```python
from build123d import *

# Parameters (mm, degrees)
SKETCH001_W   = 141
SKETCH001_H   = 55
PAD_DEPTH     = 3.6
SKETCH002_R   = 5
SKETCH002_R_2 = 1.6
PAD001_DEPTH  = 2
SKETCH003_R   = 1
POCKET_DEPTH  = 1.601


with BuildPart() as part:
    # Sketch001 → Pad (new body)
    with BuildSketch(Plane.XY):
        with BuildLine():
            Line((0, -3), (141, -3))
            ThreePointArc((141, -3), (143.12132, -2.12132), (144, 0))
            Line((144, 0), (144, 55))
            ThreePointArc((144, 55), (143.12132, 57.12132), (141, 58))
            Line((141, 58), (0, 58))
            ThreePointArc((0, 58), (-2.12132, 57.12132), (-3, 55))
            Line((-3, 55), (-3, 0))
            ThreePointArc((-3, 0), (-2.12132, -2.12132), (0, -3))
        make_face()
        with Locations((70.5, 27.5)):
            Rectangle(SKETCH001_W, SKETCH001_H, mode=Mode.SUBTRACT)
    extrude(amount=PAD_DEPTH)

    # Sketch002 → Pad001 (join)
    with BuildSketch(Plane.XY):
        with Locations((3.19, 34.92)):
            Circle(SKETCH002_R)
        with Locations((3.19, 34.92)):
            Circle(SKETCH002_R_2, mode=Mode.SUBTRACT)
        with Locations((3.19, 4.44)):
            Circle(SKETCH002_R)
        with Locations((3.19, 4.44)):
            Circle(SKETCH002_R_2, mode=Mode.SUBTRACT)
        with Locations((137.81, 4.44)):
            Circle(SKETCH002_R)
        with Locations((137.81, 4.44)):
            Circle(SKETCH002_R_2, mode=Mode.SUBTRACT)
        with Locations((137.81, 34.92)):
            Circle(SKETCH002_R)
        with Locations((137.81, 34.92)):
            Circle(SKETCH002_R_2, mode=Mode.SUBTRACT)
    extrude(amount=PAD001_DEPTH)

    # Sketch003 → Pocket (cut, through all)
    with BuildSketch(Plane.XY.offset(2)):
        with Locations((0, 55)):
            Circle(SKETCH003_R)
        with Locations((141, 55)):
            Circle(SKETCH003_R)
        Circle(SKETCH003_R)
        with Locations((141, 0)):
            Circle(SKETCH003_R)
    extrude(amount=POCKET_DEPTH, mode=Mode.SUBTRACT)


solid = part.part
```
Work out the finished part from the listing and answer in its coordinate system (mm). A direction names the side the tool comes from. Give positions to 0.01 mm unless a question says otherwise; leave off trailing zeros. Order: outer loops, then holes, each group sorted by start corner. A loop starts at its lowest first (then second) coordinate and runs counter-clockwise, first axis right, second up.
1. This flat-tipped pin is pushed along its axis until it touches: P1, Ø5, axis at x = 3.19, y = 34.92, coming from the +Z side. Where does it stop, or does it pass through?
Result sheet:
P1: stops at z = 2
2. The mould has two halves that part along X. Classify faces 1 (the flat face through (-3, 28, 2)), 2 (the flat face through (144, 27, 2)), 3 (the flat face through (70, 0, 2)), 4 (the flat face through (5, 35, 2)): released by +X, released by -X, zero draft, split by the parting line, or undercut.
Result sheet:
face 1: released by -X
face 2: released by +X
face 3: undercut
face 4: undercut
3. Section B-B, the plane y = 14 is taken. Determine the outline of the cut face in (x, z), and give its area (3 significant figures).
Result sheet:
outline: (-3, 0) - (0, 0) - (0, 3.6) - (-3, 3.6) - close; (141, 0) - (144, 0) - (144, 3.6) - (141, 3.6) - close
area: 21.6 mm2
4. For faces 5 (the cylindrical face through (143.1, -2.14, 1.77)), 6 (the flat face through (5, 5, 2)), 7 (the flat face through (70, 55, 2)), determine the directions among +Z, -Z, +X, -X, +Y, -Y from which every point of the face is accessible in a straight line to the end or side of a thin tool.
Result sheet:
face 5: +Z, -Z, +X, -Y
face 6: +Z
face 7: +Z, -Z
5. Section C-C, the plane x = 34.5 is taken. Determine the outline of the cut face in (y, z), and give its area (3 significant figures).
Result sheet:
outline: (-3, 0) - (0, 0) - (0, 3.6) - (-3, 3.6) - close; (55, 0) - (58, 0) - (58, 3.6) - (55, 3.6) - close
area: 21.6 mm2
6. Section A-A, the plane x = 3.19 is taken. Determine the outline of the cut face in (y, z).
Result sheet:
outline: (-3, 0) - (2.84, 0) - (2.84, 2) - (0, 2) - (0, 3.6) - (-3, 3.6) - close; (6.04, 0) - (9.44, 0) - (9.44, 2) - (6.04, 2) - close; (29.92, 0) - (33.32, 0) - (33.32, 2) - (29.92, 2) - close; (36.52, 0) - (39.92, 0) - (39.92, 2) - (36.52, 2) - close; (55, 0) - (58, 0) - (58, 3.6) - (55, 3.6) - close
7. Straight lines are drawn through the part: L1, parallel to Y at x = 137.81, z = 1.6; L2, parallel to Y at x = 121, z = 0.5; L3, parallel to X at y = 34, z = 1.05. For each, find the intervals that lie inside material, in ascending order.
Result sheet:
L1: y = -3 to 2.84, 6.04 to 9.44, 29.92 to 33.32, 36.52 to 39.92, 55 to 58
L2: y = -3 to 0, 55 to 58
L3: x = -3 to 1.88, 4.5 to 8.1, 132.9 to 136.5, 139.12 to 144
8. Section D-D, the plane y = 4.44 is taken. Determine the outline of the cut face in (x, z).
Result sheet:
outline: (-3, 0) - (1.59, 0) - (1.59, 2) - (0, 2) - (0, 3.6) - (-3, 3.6) - close; (4.79, 0) - (8.19, 0) - (8.19, 2) - (4.79, 2) - close; (132.81, 0) - (136.21, 0) - (136.21, 2) - (132.81, 2) - close; (139.41, 0) - (144, 0) - (144, 3.6) - (141, 3.6) - (141, 2) - (139.41, 2) - close
